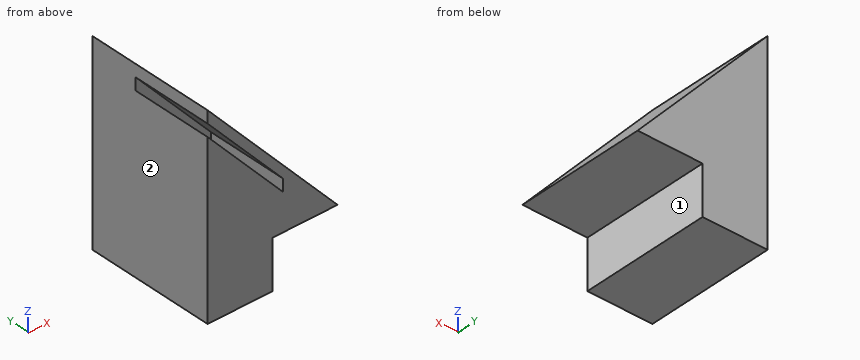
from build123d import *

# Parameters (mm, degrees)
F1_DEPTH = 101.6
F3_DEPTH = 63.5


with BuildPart() as f1:
    # F0 (on Front) → F1 (new body)
    with BuildSketch(Plane.XZ):
        Polygon((-61.3276321992, 97.2424396313), (-61.3276321992, -55.1575603687), (-10.5276321992, -55.1575603687), (-10.5276321992, -17.0575603687), (40.2723678008, -17.0575603687), align=None)
    extrude(amount=F1_DEPTH)

    # F2 (on face) → F3 (cut)
    with BuildSketch(Plane.XZ.offset(101.6)):
        Polygon((-61.3276321992, 87.6844239344), (-61.3276321992, 78.1264082375), (-2.2656869272, 11.6817198065), (-2.2656869272, 21.2397355034), align=None)
    extrude(amount=-F3_DEPTH, mode=Mode.SUBTRACT)


solid = f1.part
Geometry: final body of the model. Coordinates: model frame, mm. Face numbers are marked on the shaded views. A direction names the side the tool comes from. Give positions to 0.01 mm unless a question says otherwise; leave off trailing zeros. Loops run counter-clockwise (first coordinate to the right, second up) from the corner with the lowest first, then second, coordinate; pieces in that order, holes last. Notation, with made-up numbers: (15.25, -13.75) - (72.25, -13.75) arc R29 cw to (72.25, 15.25) - close; hole circle Ø2 at (4.5, 16.25). An arc over 180 degrees is marked (long way). Answer as CSV lines item,"result". Start each with the question number.
1. Section D-D, the plane y = -86.5. Return loops of the section in (x, z), plus the area to 3 significant figures.
2. Pin query (flat end, axial travel): P1, Ø8, axis at y = -27.5, z = -3, coming from the +X side; P2, Ø5, axis at x = -11, y = -90.5, coming from the +Z side; P3, Ø2, axis at y = -50, z = 17, coming from the +X side. Return the tip coordinate at first contact, or that it passes through.
3. Section A-A, the plane y = -29.5. Return loops of the section in (x, z), plus the area to 3 significant figures.
4. Section C-C, the plane x = -24. Return loops of the section in (y, z), plus the area to 3 significant figures.
5. Section B-B, the plane z = 31.5. Return loops of the section in (x, y), plus the area to 3 significant figures.
6. Reachability of the marked faces 1 and 2 from +Z, -Z, +X, -X, +Y, -Y: full face, straight path, thin tool, end or side. Return the list, or none.
7. Ray query, L1, parallel to Y at x = -6.5, z = 21; L2, parallel to X at y = -84, z = 48.5; L3, parallel to Z at x = -26, y = -80.5. Return the intervals inside material, ascending.
Answers:
1,outline,"(-61.33, -55.16) - (-10.53, -55.16) - (-10.53, -17.06) - (40.27, -17.06) - (-61.33, 97.24) - (-61.33, 87.68) - (-2.27, 21.24) - (-2.27, 11.68) - (-61.33, 78.13) - close"
1,area,"7,180 mm2"
2,P1,"stops at x = 31.33"
2,P2,"stops at z = 43.44"
2,P3,"stops at x = 10.89"
3,outline,"(-61.33, -55.16) - (-10.53, -55.16) - (-10.53, -17.06) - (40.27, -17.06) - (-61.33, 97.24) - close"
3,area,"7,740 mm2"
4,outline,"(-101.6, -55.16) - (0, -55.16) - (0, 55.25) - (-101.6, 55.25) - (-101.6, 45.69) - (-38.1, 45.69) - (-38.1, 36.13) - (-101.6, 36.13) - close"
4,area,"10,600 mm2"
5,outline,"(-61.33, -101.6) - (-19.88, -101.6) - (-19.88, -38.1) - (-11.39, -38.1) - (-11.39, -101.6) - (-2.89, -101.6) - (-2.89, 0) - (-61.33, 0) - close"
5,area,"5,400 mm2"
6,face 1,"-Z, +X, +Y, -Y"
6,face 2,"+Z, -Z, -X, +Y, -Y"
7,L1,"y = -38.1 to 0"
7,L2,"x = -61.33 to -34.99, -26.5 to -18"
7,L3,"z = -55.16 to 38.38, 47.94 to 57.5"
